from build123d import *

# Parameters (mm, degrees)
F3_R = 6.35
F4_R = 6.35
F5_R = 6.35


with BuildPart() as f2:
    # F2: sweep along a path in F1
    with BuildLine(Plane.XZ) as f2_path:
        Line((0, 0), (-400.05, 0))
    # F0 (on Right) → F2 (sweep)
    with BuildSketch(Plane.YZ):
        with BuildLine():
            ThreePointArc((107.7558518291, 0), (15.6808518291, -8.0168287935), (-76.3941481709, 0))
            Line((-76.3941481709, 0), (-76.9428730772, -3.1272233654))
            ThreePointArc((-76.9428730772, -3.1272233654), (15.6808518291, -11.1918287935), (108.3045767353, -3.1272233654))
            Line((108.3045767353, -3.1272233654), (107.7558518291, 0))
        make_face()
    sweep(path=f2_path.line)

    # F3
    f3_edges = [f2.edges().sort_by_distance(p)[0] for p in [
        (-400.05, -76.668511, -1.563612),
    ]]
    fillet(f3_edges, radius=F3_R)

    # F4
    f4_edges = [f2.edges().sort_by_distance(p)[0] for p in [
        (-400.05, 108.030214, -1.563612),
        (0, 108.030214, -1.563612),
    ]]
    fillet(f4_edges, radius=F4_R)

    # F5
    f5_edges = [f2.edges().sort_by_distance(p)[0] for p in [
        (0, -76.668511, -1.563612),
    ]]
    fillet(f5_edges, radius=F5_R)


solid = f2.part
Here's how the part is built. I have some questions about the finished solid (model axes, mm). Coordinates: 2 decimals unless noted, no trailing zeros. Order: outer loops, then holes, each group sorted by start corner. A loop starts at its lowest first (then second) coordinate and runs counter-clockwise, first axis right, second up. Notation, with made-up numbers: M -39.75,-29 L -22.75,-29 A26 ccw -22.75,10 Z; hole C -14,-33.75 d2. An arc over 180 degrees is marked long. Answer as CSV lines item,"result". Start each with the question number.
1. I want a section at C-C, the plane y = -16.5. Write out the boundary of the cut face in (x, z).
2. I want a section at B-B, the plane x = -300. Write out the boundary of the cut face in (y, z), and give its area (3 significant figures).
3. We'd pull the mould along Y, two halves only. Please class faces 1 (the cylindrical face through (-202.83, 16.98, -11.19)), 2 (the flat face through (-400.05, 15.3, -8.4)), 3 (the cylindrical face through (-202.825, 16.976, -8.015)): released by +Y, released by -Y, zero draft, split by the parting line, or undercut.
4. I need wall thicknesses on line 1 (Z direction, x = -357, y = -56); line 2 (Z direction, x = -186, y = -58.5). Which ranges of each line are inside material? Lowest first, please. Write a range as [from, to].
Recorded:
1,outline,"M -400.05,-10.22 L 0,-10.22 L 0,-7.04 L -400.05,-7.04 Z"
2,outline,"M -76.94,-3.13 A535.93 ccw 108.3,-3.13 L 107.76,0 A532.76 cw -76.39,0 Z"
2,area,"589 mm2"
3,face 1,"split by the parting line"
3,face 2,"zero draft"
3,face 3,"undercut"
4,line 1,"z = [-6.38, -3.17]"
4,line 2,"z = [-6.03, -2.83]"
